Could you check a few things on this model? Use its own coordinates, in mm. Round coordinates to 2 decimals unless told otherwise and drop trailing zeros. Loops run counter-clockwise (first coordinate to the right, second up) from the corner with the lowest first, then second, coordinate; pieces in that order, holes last. Notation, with made-up numbers: (-29.5, 10.25) -> (-7.5, 10.25) arc R14 cw to (-7.5, 31.25) -> close; hole circle Ø4 at (29.25, 22.5). An arc over 180 degrees is marked (long way). Write each question's results on one line, items separated by ' | '. Start each with the question number.
1) Imagine slicing it at A-A, the plane z = 10. List the corners of the cut face in (x, y) for me, plus the area to 3 significant figures.
2) For P1, Ø2, axis at x = -9, z = 9.5, coming from the +Y side; P2, Ø5, axis at y = -5, z = 5, coming from the +X side; P3, Ø6, axis at x = 6, z = 4.5, coming from the -Y side; P4, Ø3, axis at y = 6.5, z = 8, coming from the +X side, each with a flat end and sliding along its axis, tell me the tip position at first contact or that it passes through.
3) If I drill on probe 1 along Z at (x, y) = (-10.5, 5.75); probe 2 along Y at (x, z) = (-8.25, 3.5); probe 3 along X at (y, z) = (3.5, 4.25), over which ranges is the centre line in solid material (lowest first)?
4) Imagine slicing it at B-B, the plane z = 8. List the corners of the cut face in (x, y) for me.
from build123d import *

# Parameters (mm, degrees)
SKETCH_R          = 12.5
PAD_DEPTH         = 3
SPHERE_ANGLE      = 180
SPHERE_ROLL_ANGLE = 90
FILLET_R          = 2


with BuildPart() as base_pad:
    # Sketch → Pad (new body)
    with BuildSketch(Plane.XY):
        Circle(SKETCH_R)
    extrude(amount=PAD_DEPTH)


with BuildPart() as fillet_body:
    # Sphere → Sphere (revolve)
    with BuildSketch(Plane.XZ):
        with BuildLine():
            ThreePointArc((0, -10), (10, 0), (0, 10))
            Line((0, 10), (0, -10))
        make_face()
    revolve(axis=Axis((0, 0, 0), (0, 0, 1)), revolution_arc=SPHERE_ANGLE)


with BuildPart() as fillet_body_1:
    # Sphere roll: moved
    add(fillet_body.part.rotate(Axis((0, 0, 0), (1, 0, 0)), SPHERE_ROLL_ANGLE))


with BuildPart() as fillet_body_2:
    # Sphere placement: moved
    add(fillet_body_1.part.moved(Location((0, 0, 2.4))))

    # Fusion: union Base-pad
    add(base_pad.part)

    # Fillet
    fillet_edges = [fillet_body_2.edges().sort_by_distance(p)[0] for p in [
        (0, -9.981984, 3),
    ]]
    fillet(fillet_edges, radius=FILLET_R)


solid = fillet_body_2.part
Checked values:
1) outline: circle Ø13 at (0, 0) | area: 133 mm^2
2) P1: through | P2: x = 12 | P3: y = -12.03 | P4: x = 7.06
3) probe 1: 0 to 3 | probe 2: -6.32 to 6.32 | probe 3: -9.22 to 9.22
4) outline: circle Ø16.57 at (0, 0)
